Geometry check sheet. Reference: the model listing, model coordinates, mm. A direction names the side the tool comes from. Coordinates: 2 decimals unless noted, no trailing zeros. Order: outer loops, then holes, each group sorted by start corner. A loop starts at its lowest first (then second) coordinate and runs counter-clockwise, first axis right, second up. Notation, with made-up numbers: (11, 15) - (20, 15) arc R9 ccw to (20, 30) - close; hole circle Ø6 at (-36, 56). An arc over 180 degrees is marked (long way). One line per item, written item: value. Start each with the question number.
```python
from build123d import *

# Parameters (mm, degrees)
F0_R     = 66.641501
F0_R_2   = 9.968602
F0_R_3   = 8.169594
F0_R_4   = 10.130103
F1_DEPTH = 150


with BuildPart() as f1:
    # F0 (on Front) → F1 (new body)
    with BuildSketch(Plane.XZ):
        Circle(F0_R)
        with BuildLine():
            ThreePointArc((-47.21239, -19.541254), (-50.009162, -13.621133), (-52.03151, -7.393784))
            Line((-52.03151, -7.393784), (-34.136722, -7.393784))
            Line((-34.136722, -7.393784), (-21.011824, -7.393784))
            Line((-21.011824, -7.393784), (-8.125476, -7.393784))
            Line((-8.125476, -7.393784), (5.238163, -7.393784))
            Line((5.238163, -7.393784), (14.783629, -7.393784))
            Line((14.783629, -7.393784), (23.911529, -7.393784))
            Line((23.911529, -7.393784), (32.681515, -7.393784))
            Line((32.681515, -7.393784), (44.854218, -7.393784))
            Line((44.854218, -7.393784), (44.854218, -15.515085))
            ThreePointArc((44.854218, -15.515085), (43.897568, -17.550039), (42.852925, -19.541254))
            ThreePointArc((42.852925, -19.541254), (38.288746, -26.426826), (32.681515, -32.493274))
            ThreePointArc((32.681515, -32.493274), (28.469498, -35.978188), (23.911529, -38.996572))
            ThreePointArc((23.911529, -38.996572), (19.451177, -41.334676), (14.783629, -43.225568))
            ThreePointArc((14.783629, -43.225568), (10.066868, -44.623512), (5.238163, -45.564626))
            ThreePointArc((5.238163, -45.564626), (-1.43737, -46.096762), (-8.125476, -45.757446))
            ThreePointArc((-8.125476, -45.757446), (-14.673168, -44.56238), (-21.011824, -42.532135))
            ThreePointArc((-21.011824, -42.532135), (-27.853806, -39.239377), (-34.136722, -34.975583))
            ThreePointArc((-34.136722, -34.975583), (-41.440477, -27.907292), (-47.21239, -19.541254))
        make_face(mode=Mode.SUBTRACT)
        with BuildLine():
            ThreePointArc((-11.232171, 13.509632), (-8.938658, 10.432505), (-8.125476, 6.681819))
            ThreePointArc((-8.125476, 6.681819), (-25.42498, 2.931132), (-11.232171, 13.509632))
        make_face(mode=Mode.SUBTRACT)
        with Locations((-33.41883, 39.852273)):
            Circle(F0_R_2, mode=Mode.SUBTRACT)
        with Locations((2.872223, 5.739587)):
            Circle(F0_R_3, mode=Mode.SUBTRACT)
        with Locations((25.047079, 39.852273)):
            Circle(F0_R_4, mode=Mode.SUBTRACT)
    extrude(amount=F1_DEPTH)


solid = f1.part
```
Q1. Cross-section at C-C, the plane z = 0. Enter the section's corners in (x, y).
Q2. Cross-section at B-B, the plane y = -18. Enter the section's corners in (x, z).
Q3. Release check for a two-part mould opening along X. For faces 1 (the cylindrical face through (-49.975, -73.95, -13.706)), 2 (the cylindrical face through (63.564, -73.95, 20.017)), 3 (the flat face through (14, -150, 1)) record: released by +X, released by -X, zero draft, split by the parting line, or undercut.
Q4. Gauge pin test, flat ends, axial feed: P1, Ø5, axis at x = -20.5, z = -40, coming from the +Y side (3 decimals); P2, Ø5, axis at y = -99.5, z = 28, coming from the +X side; P3, Ø8, axis at x = -23, z = -52, coming from the +Y side; P4, Ø10, axis at x = 43.5, y = -19, coming from the +Z side. Record the tip position at first contact, or that the pin passes through.
Q5. Material ranges on probe 1 along Z at (x, y) = (-25.5, -136.5); probe 2 along Z at (x, y) = (16.5, -19); probe 3 along Z at (x, y) = (-4, -119.5), recorded low to high.
Q6. Cross-section at D-D, the plane x = -58. Enter the section's corners in (y, z).
Q7. Set-up check for faces 4 (the cylindrical face through (-14.583, -73.95, -44.585)), 5 (the flat face through (14, 0, 1)): record each of +Z, -Z, +X, -X, +Y, -Y from which the full face is reachable in a straight line by a thin tool's end or side.
Q8. Cross-section at A-A, the plane x = 0. Enter the section's corners in (y, z), and give its area (3 significant figures).
Check result:
1. outline: (-66.64, -150) - (-23.29, -150) - (-23.29, 0) - (-66.64, 0) - close; (-11.07, -150) - (-2.94, -150) - (-2.94, 0) - (-11.07, 0) - close; (8.69, -150) - (66.64, -150) - (66.64, 0) - (8.69, 0) - close
2. outline: circle Ø133.28 at (0, 0); hole (-52.03, -7.39) arc R51.46 ccw to (-47.21, -19.54) arc R51.46 ccw to (-34.14, -34.98) arc R51.46 ccw to (-21.01, -42.53) arc R51.46 ccw to (-8.13, -45.76) arc R51.46 ccw to (5.24, -45.56) arc R51.46 ccw to (14.78, -43.23) arc R51.46 ccw to (23.91, -39) arc R51.46 ccw to (32.68, -32.49) arc R51.46 ccw to (42.85, -19.54) arc R51.46 ccw to (44.85, -15.52) - (44.85, -7.39) - close; hole circle Ø19.94 at (-33.42, 39.85); hole (-11.23, 13.51) arc R9.06 ccw (long way) to (-8.13, 6.68) arc R9.06 ccw to start; hole circle Ø16.34 at (2.87, 5.74); hole circle Ø20.26 at (25.05, 39.85)
3. face 1: undercut
3. face 2: split by the parting line
3. face 3: zero draft
4. P1: passes through
4. P2: stops at x = 61.57
4. P3: stops at y = 0
4. P4: stops at z = 54.4
5. probe 1: z = -61.57 to -40.51, -7.39 to 3.1, 10.26 to 33.8, 45.91 to 61.57
5. probe 2: z = -64.57 to -42.59, -7.39 to 34.41, 45.29 to 64.57
5. probe 3: z = -66.52 to -46.07, -7.39 to 1.32, 10.16 to 66.52
6. outline: (-150, -32.82) - (0, -32.82) - (0, 32.82) - (-150, 32.82) - close
7. face 4: +Y, -Y
7. face 5: +Z, -Z, +X, -X, +Y
8. outline: (-150, -66.64) - (0, -66.64) - (0, -46.06) - (-150, -46.06) - close; (-150, -7.39) - (0, -7.39) - (0, -1.91) - (-150, -1.91) - close; (-150, 13.39) - (0, 13.39) - (0, 66.64) - (-150, 66.64) - close
8. area: 11,900 mm2
